Autodesk Fusion 360 part; units mm, degrees
sketch "Skizze1" plane through (0, 0, 0) normal (0, 1, 0) x (1, 0, 0)
  line L0 (0, 0) -> (-75.0363, 0)
  line L1 (-90.0714, -21.4723) -> (-60.8666, -101.7116)
  line L2 (0, 0) -> (0, -8)
  line L3 (0, -8) -> (-75.0363, -8)
  line L4 (-82.5538, -18.7362) -> (-53.3491, -98.9755)
  line L5 (-44.3205, -99.7654) -> (-17.3205, -53)
  line L6 (-17.3205, -53) -> (0, -63)
  line L7 (0, -63) -> (-5.5, -72.5263)
  line L8 (-5.5, -72.5263) -> (-8.9641, -70.5263)
  line L9 (-8.9641, -70.5263) -> (-5.4641, -64.4641)
  line L10 (-5.4641, -64.4641) -> (-12.3923, -60.4641)
  line L11 (-12.3923, -60.4641) -> (-37.3923, -103.7654)
  arc A0 (-53.3491, -98.9755) -> (-44.3205, -99.7654) centre (-48.6506, -97.2654) ccw
  arc A1 (-60.8666, -101.7116) -> (-37.3923, -103.7654) centre (-48.6506, -97.2654) ccw
  arc A2 (-75.0363, 0) -> (-90.0714, -21.4723) centre (-75.0363, -16) ccw
  arc A3 (-75.0363, -8) -> (-82.5538, -18.7362) centre (-75.0363, -16) ccw
  dimension "d3" = 8
  dimension "d4" = 8
  dimension "d5" = 8
  dimension "d7" = 30
  dimension "d8" = 4
  dimension "d10" = 4
  dimension "d11" = 8
  dimension "d12" = 7
  dimension "d19" = 70
  dimension "d20" = 50
  dimension "d21" = 5
  dimension "d23" = 8
  dimension "d24" = 45
extrude "Extrusion1" add sketch "Skizze1" along normal mid plane 60
fillet "Abrundung1" radius 10 2 edges at (0, 30, 4) (0, -30, 4)
fillet "Abrundung2" radius 5 2 edges at (-17.3205, 0, 53) (0, 0, 63)
sketch "Skizze2" plane through (-86.4361, 0, 31.4602) normal (-0.9397, 0, 0.342) x (0, -1, 0)
  line L0 (30, 74.7601) -> (-30, 74.7601)
  line L1 (-30, 74.7601) -> (-30, -10.6288)
  line L2 (-30, -10.6288) -> (30, -10.6288)
  line L3 (30, -10.6288) -> (30, 74.7601)
  line L4 (37, 74.7601) -> (69, 74.7601) construction
  line L5 (40.6572, -10.6288) -> (65.6572, -10.6288) construction
  line L6 (0, 61.418) -> (-15, 53.4128)
  line L7 (-15, 53.4128) -> (0, 45.4076)
  line L8 (0, 45.4076) -> (15, 53.4128)
  line L9 (15, 53.4128) -> (0, 61.418)
  line L10 (0, 95.9999) -> (0, -24.4616) construction
  line L11 (-15, 32.0656) -> (0, 40.0708)
  line L12 (15, 32.0656) -> (0, 24.0604)
  line L13 (0, 24.0604) -> (-15, 32.0656)
  line L14 (0, 40.0708) -> (15, 32.0656)
  line L15 (-15, 10.7184) -> (0, 18.7236)
  line L16 (15, 10.7184) -> (0, 2.7132)
  line L17 (0, 18.7236) -> (15, 10.7184)
  line L18 (0, 2.7132) -> (-15, 10.7184)
  line L19 (57.2523, 53.4128) -> (36.8368, 53.4128) construction
  line L20 (40.2669, 10.7184) -> (51.2669, 10.7184) construction
  line L21 (43.1326, 32.0656) -> (76.5646, 32.0656) construction
  line L22 (-30, 110.8277) -> (-30, 88.3059) construction
  line L23 (30, 114.6963) -> (30, 87.6508) construction
  line L24 (-15, 108.062) -> (-15, 86.5063) construction
  line L25 (15, 103.3946) -> (15, 87.227) construction
  line L26 (38.9734, 64.0864) -> (51.9734, 64.0864) construction
  line L27 (38.9734, 58.7496) -> (51.9734, 58.7496) construction
  line L28 (39, 61.418) -> (48, 61.418) construction
  line L29 (38.4081, 40.0708) -> (47.4081, 40.0708) construction
  line L30 (37.9929, 37.4024) -> (54, 37.4024) construction
  line L31 (38.8043, 42.7392) -> (51.8043, 42.7392) construction
  line L32 (38.9581, 21.392) -> (51.9581, 21.392) construction
  line L33 (38.4081, 18.7236) -> (47.4081, 18.7236) construction
  line L34 (40.1572, 16.0552) -> (53.1572, 16.0552) construction
sketch "Skizze3" plane through (0, 0, 0) normal (0, 0, -1) x (1, 0, 0)
  line L0 (-10, 30) -> (-75.0363, 30)
  line L1 (-75.0363, 30) -> (-75.0363, -30)
  line L2 (-75.0363, -30) -> (-10, -30)
  line L3 (-37.5181, 22.5) -> (-15.0181, 0)
  line L4 (-15.0181, 0) -> (-37.5181, -22.5)
  line L5 (-37.5181, -22.5) -> (-60.0181, 0)
  line L6 (-60.0181, 0) -> (-37.5181, 22.5)
  line L7 (20.4049, 0) -> (39.4049, 0) construction
  line L8 (22.3322, 30) -> (39.3616, 30) construction
  line L9 (19.3322, -30) -> (41.3322, -30) construction
  line L10 (-37.5181, 48.9997) -> (-37.5181, 36.9997) construction
  line L11 (-75.0363, 50.8097) -> (-75.0363, 32.3583) construction
  line L12 (0, 53.6395) -> (0, 35.107) construction
  arc A0 (0, 20) -> (-10, 30) centre (-10, 20) ccw
  arc A1 (-10, -30) -> (0, -20) centre (-10, -20) ccw
  line L13 (0, -20) -> (0, 20)
  dimension "d82" = 7.5
sketch "Skizze4" plane through (0, 0, 0) normal (0, 1, 0) x (1, 0, 0)
  line L0 (-7.5, -75.9904) -> (-24.8205, -65.9904)
  line L1 (-24.8205, -65.9904) -> (-17.3205, -53)
  line L2 (-17.3205, -53) -> (0, -63)
  line L3 (0, -63) -> (-7.5, -75.9904)
  line L4 (-4.3301, -60.5) -> (-12.9904, -55.5)
  line L5 (-5.5, -72.5263) -> (-2.5, -67.3301)
  line L6 (-19.8205, -57.3301) -> (-44.3205, -99.7654)
  dimension "d68" = 15
extrude "Extrusion2" cut sketch "Skizze4" along normal mid plane 20
fillet "Abrundung3" radius 4 2 edges at (-21.3564, 10, 67.9904) (-21.3564, -10, 67.9904)
sketch "Skizze5" plane through (16.8875, 0, 9.75) normal (0.866, 0, 0.5) x (0, 1, 0)
  line L0 (30, 58.5596) -> (30, 108.5596)
  line L1 (30, 108.5596) -> (-30, 108.5596)
  line L2 (-30, 108.5596) -> (-30, 58.5596)
  line L3 (18.75, 89.0596) -> (0, 103.6846)
  line L4 (0, 103.6846) -> (-18.75, 89.0596)
  line L5 (-18.75, 89.0596) -> (0, 74.4346)
  line L6 (0, 74.4346) -> (18.75, 89.0596)
  line L7 (18.75, 89.0596) -> (-18.75, 89.0596) construction
  line L8 (0, 103.6846) -> (0, 74.4346) construction
  line L9 (0, 132.1709) -> (0, 54.7397)
  line L10 (57, 89.0596) -> (43, 89.0596) construction
  line L11 (41.8287, 108.5596) -> (56.8287, 108.5596) construction
  line L12 (41.1202, 69.5596) -> (58.1202, 69.5596) construction
  line L13 (10, 58.5596) -> (30, 58.5596)
  line L14 (15, 145.9398) -> (15, 132.9398) construction
  line L15 (22.5, 142.6003) -> (22.5, 134.6003) construction
  line L16 (42, 103.6846) -> (64, 103.6846) construction
  line L17 (42, 98.8096) -> (60, 98.8096) construction
  line L18 (18.75, 141.5724) -> (18.75, 135.5724) construction
  line L19 (10, 65.5596) -> (10, 58.5596)
  line L20 (-10, 58.5596) -> (-10, 65.5596)
  arc A0 (-6, 69.5596) -> (-10, 65.5596) centre (-6, 65.5596) ccw
  arc A1 (10, 65.5596) -> (6, 69.5596) centre (6, 65.5596) ccw
  line L21 (-6, 69.5596) -> (6, 69.5596)
  line L22 (-30, 58.5596) -> (-10, 58.5596)
  point P0 (0, 89.0596)
extrude "Extrusion3" cut sketch "Skizze5" against normal up to surface (8 mm away) contours L4 L5 L9 | L3 L6 L9
extrude "Extrusion4" cut sketch "Skizze3" against normal up to surface (8 mm away) contours L3 L4 L5 L6
extrude "Extrusion5" cut sketch "Skizze2" against normal up to surface (8 mm away) contours L6 L7 L8 L9 | L11 L12 L13 L14 | L15 L16 L17 L18
equation "angle = 30 deg"
equation "d4 = d3"
equation "d5 = d3"
equation "d7 = angle"
equation "d8 = d3 / 2"
equation "thickness = 8 mm"
equation "d10 = d8"
equation "d11 = thickness"
equation "d12 = bracket_depth"
equation "bracket_depth = 7 mm"
equation "length = 150 mm"
equation "width = 60 mm"
equation "cable_width = 20 mm"
equation "d20 = length / 3"
equation "d24 = platform_height"
equation "platform_height = 45 mm"
equation "d26 = width / 2"
equation "d50 = 45.35489 mm / 3"
equation "d53 = 90.709781 mm / 13"
equation "d54 = d53"
equation "d56 = 90.709781 mm * 3 / 14"
equation "d62 = 57.359 mm * 3 / 13"
equation "d69 = cable_width / 2"
Input: part model. Units: mm. Frame: model coordinates. A direction names the side the tool comes from. Round coordinates to 2 decimals unless told otherwise and drop trailing zeros. Write each loop counter-clockwise with the first axis right and the second up, starting at its lowest first coordinate (ties: lowest second). Pieces come first, ordered by that corner, then holes. Notation, with made-up numbers: (30, -13) -> (56, -13) arc R20 ccw to (56, 24) -> close; hole circle Ø5 at (57, 20.5). An arc over 180 degrees is marked (long way). Answer as CSV lines item,"result".
1. Section A-A (z = 77). Return the cut outline in (x, y).
Geometry says:
outline,"(-69.86, -30) -> (-61.35, -30) -> (-61.35, -11.18) -> (-69.86, -5.72) -> close; (-69.86, 5.72) -> (-61.35, 11.18) -> (-61.35, 30) -> (-69.86, 30) -> close; (-31.18, -30) -> (-21.94, -30) -> (-21.94, -4.13) -> (-31.18, -10.05) -> close; (-31.18, 10.05) -> (-21.94, 4.13) -> (-21.94, 30) -> (-31.18, 30) -> close"
2. Reachability of faces 1 (the cylindrical face through (-20.835, 8.797, 66.975)), 2 (the flat face through (-7.21, -20.14, 71.54)), 3 (the flat face through (-26.43, -11.41, 3.94)), 4 (the flat face through (-8.88, -20.14, 62.49)), 5 (the cylindrical face through (-2.85, 26.99, 4.06)) from +Z, -Z, +X, -X, +Y, -Y: full face, straight path, thin tool, end or side. Return the list, or none.
Geometry says:
face 1,"+X"
face 2,"+Z, +Y, -Y"
face 3,"-Z"
face 4,"+Y, -Y"
face 5,"-Z, +X, +Y"
3. Contact query for flat-ended pins moving along their axis: P1, Ø6, axis at y = -4, z = 84.5, coming from the +X side; P2, Ø6, axis at x = -57, y = 4.5, coming from the -Z side; P3, Ø2, axis at y = -19.5, z = 41.5, coming from the +X side; P4, Ø18, axis at x = -32.5, y = 14, coming from the +Z side. Output: stop coordinate, or through.
Geometry says:
P1,"stops at x = -57.53"
P2,"stops at z = 0"
P3,"stops at x = -73.9"
P4,"stops at z = 108.12"
4. Section C-C (z = 92.5). Return the cut outline in (x, y).
Geometry says:
outline,"(-64.22, -30) -> (-55.71, -30) -> (-55.71, 30) -> (-64.22, 30) -> close; (-40.13, -30) -> (-30.89, -30) -> (-30.89, -10.43) -> (-40.13, -4.51) -> close; (-40.13, 4.51) -> (-30.89, 10.43) -> (-30.89, 30) -> (-40.13, 30) -> close"
5. Section D-D (x = -29). Return the cut outline in (y, z), plus the area to 3 significant figures.
Geometry says:
outline,"(-30, 0) -> (-13.98, 0) -> (-13.98, 8) -> (-30, 8) -> close; (-30, 73.23) -> (-4.47, 73.23) -> (-18.75, 86.09) -> (-15.27, 89.23) -> (-30, 89.23) -> close; (4.47, 73.23) -> (30, 73.23) -> (30, 89.23) -> (15.27, 89.23) -> (18.75, 86.09) -> close; (13.98, 0) -> (30, 0) -> (30, 8) -> (13.98, 8) -> close"
area,"811 mm^2"
6. Mould query, pull axis Z, two halves, no side actions, for faces 6 (the flat face through (-73.11, -7.6, 56.53)), 7 (the flat face through (-48.93, -11.09, 3.94)), 8 (the flat face through (-3.98, 19.86, 69.89)), 9 (the flat face through (-71.4, -0.42, 49.38)). Classes: +Z half, -Z half, draft (parallel to the pull), parting line (faces both ways), or undercut.
Geometry says:
face 6,"undercut"
face 7,"draft"
face 8,"+Z half"
face 9,"undercut"
7. Ray query, L1, parallel to X at y = -5, z = 70; L2, parallel to Z at x = -67, y = 2; L3, parallel to X at y = -2, z = 7. Return the intervals inside material, ascending. Write a range as [from, to].
Geometry says:
L1,"x = [-72.41, -63.9], [-27.14, -17.9]"
L2,"z = [0, 8], [65.89, 73.84]"
L3,"x = [-88.27, -58.02], [-17.02, 0]"
8. Section B-B (x = -55.5). Return the cut outline in (y, z).
Geometry says:
outline,"(-30, 0) -> (-4.52, 0) -> (-4.52, 8) -> (-30, 8) -> close; (-30, 93.07) -> (30, 93.07) -> (30, 108.31) -> (-30, 108.31) -> close; (4.52, 0) -> (30, 0) -> (30, 8) -> (4.52, 8) -> close"
